```python
from build123d import *

# Parameters (mm, degrees)
F1_DEPTH = 20
F2_W     = 16
F2_H     = 2
F3_DEPTH = 16
F4_R     = 1.75
F5_DEPTH = 4


with BuildPart() as f1:
    # F0 (on Front) → F1 (new body)
    with BuildSketch(Plane.XZ):
        with BuildLine():
            ThreePointArc((-8, -3.7), (0, -1.7), (8, -3.7))
            Line((8, -3.7), (8, 2.3))
            Line((8, 2.3), (-8, 2.3))
            Line((-8, 2.3), (-8, -3.7))
        make_face()
    extrude(amount=F1_DEPTH)

    # F2 (on face) → F3 (cut, through all)
    with BuildSketch(Plane.YZ.offset(8)):
        with Locations((-10.047581, -0.113725)):
            Rectangle(F2_W, F2_H)
    extrude(amount=-F3_DEPTH, mode=Mode.SUBTRACT)

    # F4 (on face) → F5 (join)
    with BuildSketch(Plane.XY.offset(2.3)):
        with Locations((-5.14, -17.108951)):
            Circle(F4_R)
        with Locations((5.14, -17.108951)):
            Circle(F4_R)
    extrude(amount=F5_DEPTH)


solid = f1.part
```
Model file for the job. Use its own axes, mm. A direction names the side the tool comes from. Give positions to 0.01 mm unless a question says otherwise; leave off trailing zeros. Write each loop counter-clockwise with the first axis right and the second up, starting at its lowest first coordinate (ties: lowest second). Pieces come first, ordered by that corner, then holes. Notation, with made-up numbers: M -18.75,-3 L -10.75,-3 A17 ccw -10.75,5 Z; hole C 76,42 d9. An arc over 180 degrees is marked long. Use a Markdown table: item, result.
1) Pull direction Y, two halves, no side cores. Call faces 4 (the cylindrical face through (-5.519, -18.817, 4.272)), 5 (the flat face through (-8, -9.9, -1.3)), 6 (the flat face through (0, -10, -1.114)): +Y half, -Y half, draft (parallel to the pull), parting line (faces both ways), or undercut.
Responses:
| item | result |
|---|---|
| face 4 | parting line |
| face 5 | draft |
| face 6 | undercut |
2) Cut at B-B (z = 0). List the corners of the cut face in (x, y).
Responses:
| item | result |
|---|---|
| outline | M -8,-20 L 8,-20 L 8,-18.05 L -8,-18.05 Z; M -8,-2.05 L 8,-2.05 L 8,0 L -8,0 Z |
3) Pin check, flat tips, straight feed: pin 1 (5 mm diameter, centred on x = -2, y = -9.5, fed in from -Z); pin 2 (5 mm diameter, centred on x = -5, y = -10.5, fed in from -Z); pin 3 (4 mm diameter, centred on x = 4.5, z = 4.5, fed in from -Y). Stop position of each tip, or through.
Responses:
| item | result |
|---|---|
| pin 1 | stops at z = -2.31 |
| pin 2 | stops at z = -3.44 |
| pin 3 | stops at y = -18.86 |
4) Cut at C-C (x = -5.14). List the corners of the cut face in (y, z), and give its area (3 significant figures).
Responses:
| item | result |
|---|---|
| outline | M -20,-2.5 L 0,-2.5 L 0,2.3 L -15.36,2.3 L -15.36,6.3 L -18.86,6.3 L -18.86,2.3 L -20,2.3 Z; hole M -18.05,-1.11 L -2.05,-1.11 L -2.05,0.89 L -18.05,0.89 Z |
| area | 77.9 mm2 |
5) Cut at D-D (y = -16.5). List the corners of the cut face in (x, z), and give its area (3 significant figures).
Responses:
| item | result |
|---|---|
| outline | M -8,-3.7 A17 cw 8,-3.7 L 8,-1.11 L -8,-1.11 Z; M -8,0.89 L 8,0.89 L 8,2.3 L 6.78,2.3 L 6.78,6.3 L 3.5,6.3 L 3.5,2.3 L -3.5,2.3 L -3.5,6.3 L -6.78,6.3 L -6.78,2.3 L -8,2.3 Z |
| area | 68.7 mm2 |
6) Cut at A-A (y = -11). List the corners of the cut face in (x, z), and give its area (3 significant figures).
Responses:
| item | result |
|---|---|
| outline | M -8,-3.7 A17 cw 8,-3.7 L 8,-1.11 L -8,-1.11 Z; M -8,0.89 L 8,0.89 L 8,2.3 L -8,2.3 Z |
| area | 42.4 mm2 |
7) Tool access for faces 1 (the flat face through (0, -18.048, 0)), 2 (the cylindrical face through (5.95, -18.66, 4.27)), 3 (the flat face through (-5, -17, 6.3)): list every direction of +Z, -Z, +X, -X, +Y, -Y with a clear straight run to the whole face (end or side of a thin tool).
Responses:
| item | result |
|---|---|
| face 1 | +X, -X |
| face 2 | +Z |
| face 3 | +Z, +X, -X, +Y, -Y |
8) Drill centre lines: line 1 (Y direction, x = -2.5, z = 0.75); line 2 (X direction, y = -17, z = 4.25); line 3 (Z direction, x = -2.75, y = -5.75). Where is each one in solid material? Low to high. Write a range as from..to.
Responses:
| item | result |
|---|---|
| line 1 | y = -20..-18.05, -2.05..0 |
| line 2 | x = -6.89..-3.39, 3.39..6.89 |
| line 3 | z = -1.92..-1.11, 0.89..2.3 |
